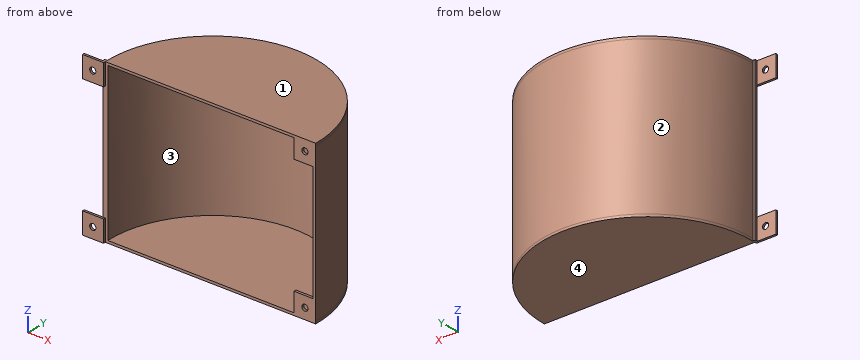
Autodesk Inventor part; units mm, degrees
ref_plane "YZ Plane" through (0, 0, 0) normal (1, 0, 0) x (0, 1, 0)
ref_plane "XZ Plane" through (0, 0, 0) normal (0, 1, 0) x (-1, 0, 0)
ref_plane "Work Plane1" through (0, 0, 65) normal (0, 0, 1) x (1, 0, 0)
sketch "Sketch1" plane through (0, 0, 65) normal (0, 0, 1) x (1, 0, 0)
  circle A0 centre (0, 0) radius 85
  line L0 (85, 0) -> (-85, 0)
  line L1 (85, 0) -> (-87, 0)
  line L2 (-87, 0) -> (-87, -2)
  line L3 (-87, -2) -> (85, -2)
  line L4 (85, -2) -> (85, 0)
  line L5 (-84.9765, -2) -> (-101.9765, -2)
  line L6 (-101.9765, -2) -> (-101.9765, -3.7)
  line L7 (-101.9765, -3.7) -> (-84.9765, -3.7)
  line L8 (-84.9765, -3.7) -> (-84.9765, -2)
  point P0 (-87, -1)
  point P1 (85, -1)
  point P2 (84.9765, -2)
  dimension "d1" = 170
  dimension "d2" = 2
  dimension "d3" = 0
  dimension "d4" = 172
  dimension "d5" = 17
  dimension "d6" = 1.7
extrude "Extrusion1" add sketch "Sketch1" against normal blind 2 contours L0 A0 | A0 L3 L0 | A0 L3 L2 L1 | L8 L7 L6 L5 L3
mirror "Mirror1" about plane through (0, 0, 0) normal (0, 0, 1) of "Extrusion1"
sketch "Sketch2" plane through (0, 0, 63) normal (0, 0, -1) x (-1, 0, 0)
  circle A0 centre (0, 0) radius 83
  arc A1 (85, 0) -> (-84.9765, -2) centre (0, 0) ccw
  line L0 (87, 0) -> (87, -2)
  line L1 (85, 0) -> (87, 0)
  line L2 (87, 0) -> (87, -2)
  line L3 (87, -2) -> (82.9759, -2)
  line L4 (84.9765, -2) -> (-84.9765, -2)
  line L5 (-82.9759, -2) -> (-84.9765, -2)
  circle A2 centre (0, 0) radius 85
  dimension "d9" = 2
  dimension "d10" = 170
extrude "Extrusion2" add sketch "Sketch2" along normal up to surface (126 mm away) contours A0 L4 A1 A2 L3 | A2 L1 L0 L3
sketch "Sketch3" plane through (-101.9765, -3.7, 65) normal (0, -1, 0) x (1, 0, 0)
  line L0 (0, 0) -> (17, 0)
  line L1 (0, 0) -> (17, 0)
  line L2 (17, 0) -> (17, -17.5)
  line L3 (17, -17.5) -> (0, -17.5)
  line L4 (0, -17.5) -> (0, 0)
  circle A0 centre (8.25, -8.75) radius 2.5
  point P0 (101.9765, -65)
  dimension "d13" = 17
  dimension "d14" = 17.5
  dimension "d15" = 5
  dimension "d16" = 8.75
  dimension "d17" = 8.75
extrude "Extrusion3" add sketch "Sketch3" against normal up to surface (1.7 mm away)
mirror "Mirror2" about plane through (0, 0, 0) normal (0, 0, 1) of "Extrusion3"
sketch "Sketch4" plane through (-84.9765, -2, 65) normal (0, -1, 0) x (1, 0, 0)
  line L0 (169.9529, 0) -> (169.9529, -130)
  line L1 (169.9529, -130) -> (152.4529, -130)
  line L2 (152.4529, -130) -> (152.4529, -112.5)
  line L3 (152.4529, -112.5) -> (169.9529, -112.5)
  line L4 (169.9529, -112.5) -> (169.9529, -130)
  circle A0 centre (161.2029, -121.25) radius 2.5
  point P0 (84.9765, -65)
  dimension "d20" = 17.5
  dimension "d21" = 17.5
  dimension "d22" = 5
  dimension "d23" = 8.75
  dimension "d24" = 8.75
extrude "Extrusion4" add sketch "Sketch4" against normal blind 2
mirror "Mirror3" about plane through (0, 0, 0) normal (0, 0, 1) of "Extrusion4"
properties part number "coupol"
Design review of the part built by this model. Coordinates are the model's own, in mm. Face numbers are marked on the shaded views. Round coordinates to 2 decimals unless told otherwise and drop trailing zeros. Write each loop counter-clockwise with the first axis right and the second up, starting at its lowest first coordinate (ties: lowest second). Pieces come first, ordered by that corner, then holes. Notation, with made-up numbers: (64, 80.5) -> (107, 80.5) arc R9 ccw to (107, 96.5) -> close; hole circle Ø11 at (-0.5, 81.25). An arc over 180 degrees is marked (long way). One line per item, written item: value. Start each with the question number.
Q1. Add section D-D (z = 38). Give the boundary of the cut face in (x, y), then the cut area to 3 significant figures.
Q2. Add section B-B (z = 56.25). Give the boundary of the cut face in (x, y).
Q3. Insertion check: P1, Ø1, axis at x = 41, z = 3.5, coming from the -Y side; P2, Ø2, axis at x = -43, z = 15, coming from the +Y side; P3, Ø0.8, axis at y = -2.5, z = 55, coming from the +X side. Each pin has a flat end and moves straight along its axis. Give the tip position at first contact, or say it passes through.
Q4. The part is to be moulded in two halves that separate along Z. For the marked faces 1, 2, 3 and 4, say which applies: pulls with the +Z half, pulls with the -Z half, needs draft (parallel to the pull), parting line crosses it, or undercut.
Q5. Add section C-C (y = 10.5). Give the boundary of the cut face in (x, z), then the cut area to 3 significant figures.
Q6. Add section A-A (x = 0). Give the boundary of the cut face in (y, z).
Q7. To check wall thickness, follow probe 1 along X at (y, z) = (-1, -56); probe 2 along Z at (x, y) = (-16, 67); probe 3 along X at (y, z) = (28.5, 18). State the ranges of each line that lie inside material, in increasing order.
Response:
1. outline: (-87, -2) -> (-82.98, -2) arc R83 cw (long way) to (82.98, -2) -> (84.98, -2) arc R85 ccw (long way) to (-85, 0) -> (-87, 0) -> close
1. area: 540 mm^2
2. outline: (-101.98, -3.7) -> (-96.23, -3.7) -> (-96.23, -2) -> (-101.98, -2) -> close; (-91.23, -3.7) -> (-84.98, -3.7) -> (-84.98, -2) -> (-82.98, -2) arc R83 cw (long way) to (83, 0) -> (78.73, 0) -> (78.73, -2) -> (84.98, -2) arc R85 ccw (long way) to (-85, 0) -> (-87, 0) -> (-87, -2) -> (-91.23, -2) -> close; (67.48, -2) -> (73.73, -2) -> (73.73, 0) -> (67.48, 0) -> close
3. P1: stops at y = 71.88
3. P2: stops at y = 73.9
3. P3: stops at x = -84.98
4. face 1: pulls with the +Z half
4. face 2: needs draft
4. face 3: undercut
4. face 4: pulls with the -Z half
5. outline: (-84.35, -65) -> (84.35, -65) -> (84.35, 63) -> (84.35, 65) -> (-84.35, 65) -> close; hole (-82.33, -63) -> (82.33, -63) -> (82.33, 63) -> (-82.33, 63) -> close
5. area: 1,180 mm^2
6. outline: (-2, -65) -> (85, -65) -> (85, 65) -> (-2, 65) -> (-2, 63) -> (83, 63) -> (83, -63) -> (-2, -63) -> close
7. probe 1: x = -87 to -82.99, 67.48 to 73.74, 78.71 to 84.99
7. probe 2: z = -65 to -63, 63 to 65
7. probe 3: x = -80.08 to -77.95, 77.95 to 80.08
